Verification items for this drawing (mm, ordinates from the low corner). A direction names the side the tool comes from. Give positions to 0.01 mm unless a question says otherwise; leave off trailing zeros. Write each loop counter-clockwise with the first axis right and the second up, starting at its lowest first coordinate (ties: lowest second). Pieces come first, ordered by that corner, then holes. Notation, with made-up numbers: (36.5, 2) -> (78.5, 2) arc R33 cw to (78.5, 40) -> close; hole circle Ø2 at (30, 46.5). An arc over 180 degrees is marked (long way). Use one line per item in the form item = value. Start each with the question number.
(1) Set-up check for the marked faces 1 and 2: record each of +Z, -Z, +X, -X, +Y, -Y from which the full face is reachable in a straight line by a thin tool's end or side.
(2) Depth check by flat-ended pin: pin 1 Ø10 at (x, z) = (824.5, 78) entering from -Y. Enter the tip coordinate at first touch or a pass-through.
(3) Section check C-C, the plane x = 965.5. Record the cut outline in (y, z), plus the area to 3 significant figures.
(4) Release check for a two-part mould opening along Y. For the marked faces 3, 4 and 5 record: pulls with the +Y half, pulls with the -Y half, needs draft (parallel to the pull), parting line crosses it, or undercut.
(5) Scan lines: L1, parallel to X at y = 726.5, z = 46; L2, parallel to Y at x = 480.5, z = 11.5. Record each from-to range of solid material in increasing order.
(6) Section check A-A, the plane z = 55.5. Record the cut outline in (x, y), plus the area to 3 significant figures.
(7) Section check B-B, the plane y = 843.5. Record the cut outline in (x, z).
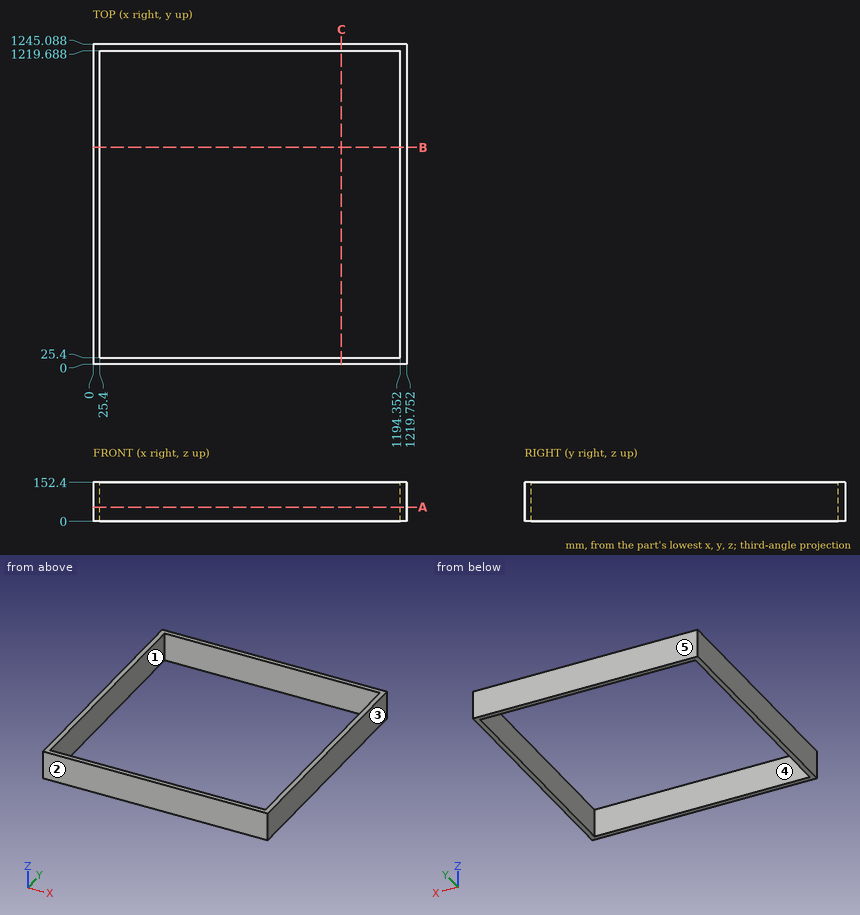
Completed:
q1.face_1 = +Z, -Z
q1.face_2 = +Z, -Z, +X, -X, -Y
q2.pin_1 = 0
q3.outline = (0, 0) -> (25.4, 0) -> (25.4, 152.4) -> (0, 152.4) -> close; (1219.69, 0) -> (1245.09, 0) -> (1245.09, 152.4) -> (1219.69, 152.4) -> close
q3.area = 7,740 mm²
q4.face_3 = needs draft
q4.face_4 = undercut
q4.face_5 = pulls with the +Y half
q5.L1 = 0 to 25.4, 1194.35 to 1219.75
q5.L2 = 0 to 25.4, 1219.69 to 1245.09
q6.outline = (0, 0) -> (1219.75, 0) -> (1219.75, 1245.09) -> (0, 1245.09) -> close; hole (25.4, 25.4) -> (1194.35, 25.4) -> (1194.35, 1219.69) -> (25.4, 1219.69) -> close
q6.area = 123,000 mm²
q7.outline = (0, 0) -> (25.4, 0) -> (25.4, 152.4) -> (0, 152.4) -> close; (1194.35, 0) -> (1219.75, 0) -> (1219.75, 152.4) -> (1194.35, 152.4) -> close
